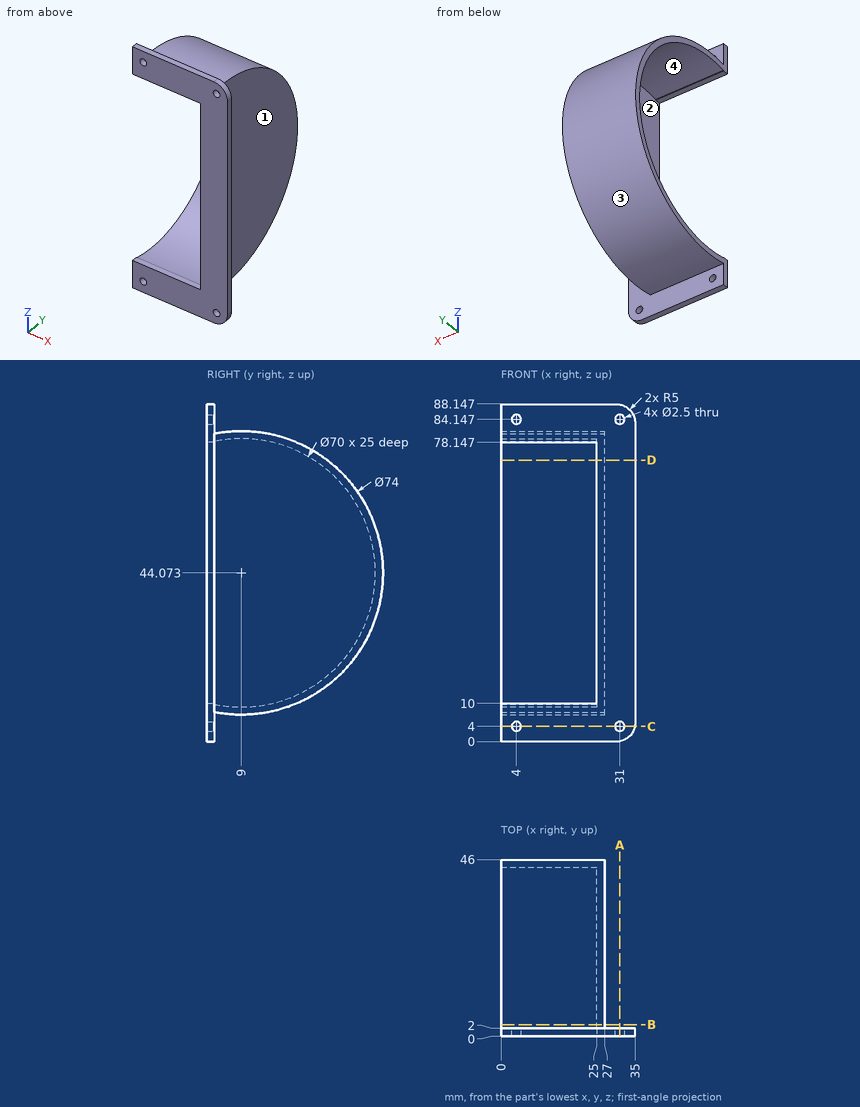
Could you check a few things on this drawing? It's one solid part, dimensions in mm from its lowest x, y, z. Give positions to 0.01 mm unless a question says otherwise; leave off trailing zeros. Write each loop counter-clockwise with the first axis right and the second up, starting at its lowest first coordinate (ties: lowest second). Pieces come first, ordered by that corner, then holes.
(1) Imagine slicing it at C-C, the plane z = 4. Write out the boundary of the cut face in (x, y).
Output values:
outline: (0, 0) - (2.75, 0) - (2.75, 2) - (0, 2) - close; (5.25, 0) - (29.75, 0) - (29.75, 2) - (5.25, 2) - close; (32.25, 0) - (34.9, 0) - (34.9, 2) - (32.25, 2) - close
(2) Will these pins go through, and if not, where does the flat tip stop? pin 1 (6 mm diameter, centred on x = 29.5, y = 8, fed in from +Z); pin 2 (2 mm diameter, centred on y = 15.5, z = 27.5, fed in from +X); pin 3 (10 mm diameter, centred on x = 19, y = 33.5, fed in from +Z); pin 4 (2 mm diameter, centred on x = 4, z = 84.15, fed in from -Y).
Output values:
pin 1: stops at z = 81.07
pin 2: stops at x = 27
pin 3: stops at z = 75.52
pin 4: passes through
(3) Thinking about a two-plate mould opening in Z: for the marked faces 1, 2, 3 and 4, which applies, pulls with the +Z half, pulls with the -Z half, needs draft (parallel to the pull), parting line crosses it, or undercut?
Output values:
face 1: needs draft
face 2: undercut
face 3: parting line crosses it
face 4: undercut
(4) Imagine slicing it at A-A, the plane x = 31. Count the separate pieces of the cut face and the enclosed holes in it, and give its area (3 significant figures).
Output values:
separate pieces: 3
enclosed holes: 0
area: 166 mm2
(5) Imagine slicing it at B-B, the plane y = 3. Write out the boundary of the cut face in (x, z) (1 decimal).
Output values:
outline: (0, 7.6) - (27, 7.6) - (27, 80.6) - (0, 80.6) - (0, 78.6) - (25, 78.6) - (25, 9.6) - (0, 9.6) - close
(6) If I drill on L1, parallel to Z at x = 4, y = 1.3; L2, parallel to Z at x = 12.25, y = 9; L3, parallel to Y at x = 30.5, z = 48, over which ranges is the centre line in solid material (lowest first)?
Output values:
L1: z = 0 to 2.75, 5.25 to 10, 78.15 to 82.9, 85.4 to 88.15
L2: z = 7.07 to 9.07, 79.07 to 81.07
L3: y = 0 to 2
(7) Imagine slicing it at D-D, the plane z = 73.5. Write out the boundary of the cut face in (x, y).
Output values:
outline: (0, 27.95) - (25, 27.95) - (25, 0) - (35, 0) - (35, 2) - (27, 2) - (27, 31.43) - (0, 31.43) - close
